Part model, mm, in its own coordinate system. A direction names the side the tool comes from. Coordinates: 2 decimals unless noted, no trailing zeros. Order: outer loops, then holes, each group sorted by start corner. A loop starts at its lowest first (then second) coordinate and runs counter-clockwise, first axis right, second up.
1) Cut at B-B (x = 34). List the corners of the cut face in (y, z).
2) Mould opens along Y. For faces 1 (the flat face through (0, -3, 0)), 2 (the cylindrical face through (66.97, 4.11, 25.76)), 3 (the flat face through (-3, 3.253, 35)) say: +Y half, -Y half, draft (parallel to the pull), parting line (faces both ways), or undercut.
3) Wall check: L1, parallel to Y at x = 0, z = 38; L2, parallel to Y at x = -15, z = 4.5; L3, parallel to X at y = -22, z = 22.5. Give the ranges that are in metal, low to high.
4) Cut at D-D (x = -27.5). List the corners of the cut face in (y, z), and give its area (3 significant figures).
5) Pin check, flat tips, straight feed: pin 1 Ø12.5 at (x, z) = (-28.5, 7.5) entering from -Y; pin 2 Ø2 at (x, z) = (16, 42.5) entering from +Y; pin 3 Ø20.5 at (x, z) = (-10.5, 13.5) entering from +Y. Stop position of each tip, or through.
6) Cut at C-C (z = 19.5). List the corners of the cut face in (x, y).
7) Cut at A-A (y = 1). List the corners of the cut face in (x, z).
8) Tool access for faces 4 (the flat face through (2, -11.525, 32)), 5 (the flat face through (-13, 13.134, 13)), 6 (the flat face through (31.5, -22.8, 50.8)), 7 (the flat face through (-20, -12, 25.4)), 8 (the flat face through (-13, -22.051, 13)): list every direction of +Z, -Z, +X, -X, +Y, -Y with a clear straight run to the whole face (end or side of a thin tool).
```python
from build123d import *

# Parameters (mm, degrees)
F1_DEPTH = 25.4
F2_R     = 30.4008834271
F3_DEPTH = 50.8
F4_R     = 23.5140896475
F5_DEPTH = 1676.4
F7_DEPTH = 25.4
F9_DEPTH = 2514.6


with BuildPart() as f1:
    # F0 (on Top) → F1 (new body)
    with BuildSketch(Plane.XY):
        with BuildLine():
            Line((24.3670896719, 13.1341721863), (-45.9093526006, 13.1341721863))
            Line((-45.9093526006, 13.1341721863), (-45.9093526006, -22.0509488136))
            Line((-45.9093526006, -22.0509488136), (27.5870569542, -22.0509488136))
            ThreePointArc((27.5870569542, -22.0509488136), (16.0056375447, -5.3709245227), (24.3670896719, 13.1341721863))
        make_face()
    extrude(amount=F1_DEPTH)

    # F2 (on Top) → F3 (join)
    with BuildSketch(Plane.XY):
        with Locations((44.5437170565, -2.9546946753)):
            Circle(F2_R)
    extrude(amount=F3_DEPTH)

    # F4 (on face) → F5 (cut)
    with BuildSketch(Plane.XY.offset(50.8)):
        with Locations((44.5437170565, -2.9546946753)):
            Circle(F4_R)
    extrude(amount=-F5_DEPTH, mode=Mode.SUBTRACT)

    # F6 (on face) → F7 (join)
    with BuildSketch(Plane.XY.offset(25.4)):
        with BuildLine():
            Line((14.7834576284, 3.2534187194), (-32.1726948023, 3.2534187194))
            Line((-32.1726948023, 3.2534187194), (-32.1726948023, -11.5247956985))
            Line((-32.1726948023, -11.5247956985), (15.375805208, -11.5247956985))
            ThreePointArc((15.375805208, -11.5247956985), (14.167225359, -4.1722599931), (14.7834576284, 3.2534187194))
        make_face()
    extrude(amount=F7_DEPTH)

    # F8 (on face) → F9 (cut)
    with BuildSketch(Plane.XZ.offset(11.5247956985)):
        Polygon((-32.1726948023, 50.8), (-32.1726948023, 25.4), (15.375805208, 50.8), align=None)
    extrude(amount=-F9_DEPTH, mode=Mode.SUBTRACT)


solid = f1.part
```
Geometry check:
1. outline: (-31.47, 0) - (-23.97, 0) - (-23.97, 50.8) - (-31.47, 50.8) - close; (18.06, 0) - (25.56, 0) - (25.56, 50.8) - (18.06, 50.8) - close
2. face 1: draft
2. face 2: undercut
2. face 3: +Y half
3. L1: y = -11.52 to 3.25
3. L2: y = -22.05 to 13.13
3. L3: x = -45.91 to 30.75, 58.33 to 68.24
4. outline: (-22.05, 0) - (13.13, 0) - (13.13, 25.4) - (3.25, 25.4) - (3.25, 27.9) - (-11.52, 27.9) - (-11.52, 25.4) - (-22.05, 25.4) - close
4. area: 931 mm2
5. pin 1: stops at y = -22.05
5. pin 2: stops at y = 9.91
5. pin 3: stops at y = 13.13
6. outline: (-45.91, -22.05) - (20.89, -22.05) arc R30.4 ccw (long way) to (18.75, 13.13) - (-45.91, 13.13) - close; hole circle Ø47.03 at (44.54, -2.95)
7. outline: (-45.91, 0) - (21.36, 0) - (21.36, 50.8) - (15.38, 50.8) - (-32.17, 25.4) - (-45.91, 25.4) - close; (67.72, 0) - (74.69, 0) - (74.69, 50.8) - (67.72, 50.8) - close
8. face 4: +Z, -X, -Y
8. face 5: +Z, -Z, -X, +Y
8. face 6: +Z, +X, -X, +Y, -Y
8. face 7: +Z, -X
8. face 8: +Z, -Z, -X, -Y
